```python
from build123d import *

# Parameters (mm, degrees)
BOSS_EXTRUDE1_DEPTH      = 6
BOSS_EXTRUDE1_DEPTH_BACK = 73
SKETCH1_W                = 60
SKETCH1_H                = 40
CUT_EXTRUDE2_DEPTH       = 10
SKETCH7_W                = 64
SKETCH7_H                = 44
SKETCH7_W_2              = 60
SKETCH7_H_2              = 40
BOSS_EXTRUDE2_DEPTH      = 11.2
SKETCH5_W                = 24
SKETCH5_H                = 3
CUT_EXTRUDE3_DEPTH       = 11.2
SKETCH8_W                = 24
SKETCH8_H                = 3
CUT_EXTRUDE4_DEPTH       = 11.2
FILLET1_R                = 5


with BuildPart() as part:
    # Sketch2 → Boss-Extrude1 (new, two sides: drawn at the far end of the back side and taken through both)
    with BuildSketch(Plane(origin=(18.941176471, 0, 0), x_dir=(0, 0, -1), z_dir=(1, 0, 0)).offset(-BOSS_EXTRUDE1_DEPTH_BACK)):
        with BuildLine():
            Line((34.764705882, 0), (-9.235294118, 0))
            add(Edge.make_bspline(
                [(-16.859042356, 8.803732274), (-16.71202536, 7.645123783), (-16.476121405, 6.983025742), (-15.665438552, 5.367344471), (-15.146819104, 4.569071681), (-14.219232142, 3.103782941), (-13.097173401, 1.202110064), (-10.958273151, -0.0861532), (-9.235294118, 0)],
                knots=[0.100936793, 0.100936793, 0.100936793, 0.100936793, 0.214701658, 0.247771225, 0.411203439, 0.4591999, 0.679739374, 1, 1, 1, 1], degree=3))
            Line((-16.859042356, 8.803732274), (-20.331201871, 8.363155033))
            Line((-20.331201871, 8.363155033), (-21.979605491, 8.153991509))
            ThreePointArc((-21.979605491, 8.153991509), (-22.976524971, 7.58463131), (-23.278855037, 6.477104328))
            Line((-23.278855037, 6.477104328), (-23.215915431, 5.981081541))
            ThreePointArc((-23.215915431, 5.981081541), (-22.646555232, 4.984162061), (-21.53902825, 4.681831995))
            Line((-21.53902825, 4.681831995), (-19.89062463, 4.890995519))
            Line((-19.89062463, 4.890995519), (-19.371936566, 4.956811088))
            add(Edge.make_bspline(
                [(-19.371936566, 4.956811088), (-19.299083809, 4.805602772), (-19.143543885, 4.495535048), (-18.861030136, 3.961180263), (-18.379944727, 3.117280646), (-17.808764188, 2.238291872), (-17.267901922, 1.360604939), (-16.505554516, 0.170581495), (-15.372861084, -1.167927692), (-13.787032793, -2.419221644), (-12.034516859, -3.186353681), (-10.648338067, -3.44710609), (-10.029136817, -3.492321417), (-9.829873201, -3.5)],
                knots=[0.220066507, 0.220066507, 0.220066507, 0.220066507, 0.244323833, 0.26858116, 0.317095812, 0.414125118, 0.511154423, 0.608183729, 0.705213035, 0.80224234, 0.899271646, 0.947786298, 0.970646745, 0.970646745, 0.970646745, 0.970646745], degree=3))
            Line((-9.829873201, -3.5), (-9.158730941, -3.5))
            Line((-9.158730941, -3.5), (34.688142706, -3.5))
            Line((34.688142706, -3.5), (35.359284966, -3.5))
            add(Edge.make_bspline(
                [(35.359284966, -3.5), (35.558548581, -3.492321417), (36.177749832, -3.44710609), (37.563928624, -3.186353681), (39.316444558, -2.419221644), (40.902272849, -1.167927692), (42.034966281, 0.170581495), (42.797313687, 1.360604939), (43.338175952, 2.238291872), (43.909356491, 3.117280646), (44.390441901, 3.961180263), (44.67295565, 4.495535048), (44.828495573, 4.805602772), (44.901348331, 4.956811088)],
                knots=[0.245720713, 0.245720713, 0.245720713, 0.245720713, 0.26858116, 0.317095812, 0.414125118, 0.511154423, 0.608183729, 0.705213035, 0.80224234, 0.899271646, 0.947786298, 0.972043625, 0.996300951, 0.996300951, 0.996300951, 0.996300951], degree=3))
            Line((44.901348331, 4.956811088), (45.420036395, 4.890995519))
            Line((45.420036395, 4.890995519), (47.068440015, 4.681831995))
            ThreePointArc((47.068440015, 4.681831995), (48.175966997, 4.984162061), (48.745327196, 5.981081541))
            Line((48.745327196, 5.981081541), (48.808266802, 6.477104328))
            ThreePointArc((48.808266802, 6.477104328), (48.505936735, 7.58463131), (47.509017256, 8.153991509))
            Line((47.509017256, 8.153991509), (45.860613636, 8.363155033))
            Line((45.860613636, 8.363155033), (42.388454121, 8.803732274))
            add(Edge.make_bspline(
                [(42.388454121, 8.803732274), (42.241437125, 7.645123783), (42.00553317, 6.983025742), (41.194850317, 5.367344471), (40.676230869, 4.569071681), (39.748643907, 3.103782941), (38.626585166, 1.202110064), (36.487684916, -0.0861532), (34.764705882, 0)],
                knots=[0.100936793, 0.100936793, 0.100936793, 0.100936793, 0.214701658, 0.247771225, 0.411203439, 0.4591999, 0.679739374, 1, 1, 1, 1], degree=3))
        make_face()
    extrude(amount=BOSS_EXTRUDE1_DEPTH + BOSS_EXTRUDE1_DEPTH_BACK)

    # Sketch1 → Cut-Extrude2 (cut)
    with BuildSketch(Plane(origin=(0, 0, 0), x_dir=(1, 0, 0), z_dir=(0, 1, 0))):
        with Locations((-13.058823529, 12.764705882)):
            Rectangle(SKETCH1_W, SKETCH1_H)
    extrude(amount=-CUT_EXTRUDE2_DEPTH, mode=Mode.SUBTRACT)

    # Sketch7 → Boss-Extrude2 (add)
    with BuildSketch(Plane.XZ.offset(3.5)):
        with Locations((-13.058823529, -12.764705882)):
            Rectangle(SKETCH7_W, SKETCH7_H)
        with Locations((-13.058823529, -12.764705882)):
            Rectangle(SKETCH7_W_2, SKETCH7_H_2, mode=Mode.SUBTRACT)
    extrude(amount=BOSS_EXTRUDE2_DEPTH)

    # Sketch5 → Cut-Extrude3 (cut)
    with BuildSketch(Plane(origin=(0, 7.29739461, 0.925955726), x_dir=(1, 0, 0), z_dir=(0, -0.9920455755956746, -0.12587921171125438))):
        with Locations((-33.058823529, 19.686118423)):
            Rectangle(SKETCH5_W, SKETCH5_H)
        with Locations((3.941176471, 19.686118423)):
            Rectangle(SKETCH5_W, SKETCH5_H)
    extrude(amount=-CUT_EXTRUDE3_DEPTH, mode=Mode.SUBTRACT)

    # Sketch8 → Cut-Extrude4 (cut)
    with BuildSketch(Plane(origin=(0, 13.957613838, -1.7710612), x_dir=(1, 0, 0), z_dir=(0, 0.9920455755956736, -0.12587921171126285))):
        with Locations((-33.058823529, 43.523881917)):
            Rectangle(SKETCH8_W, SKETCH8_H)
        with Locations((3.941176471, 43.523881917)):
            Rectangle(SKETCH8_W, SKETCH8_H)
    extrude(amount=-CUT_EXTRUDE4_DEPTH, mode=Mode.SUBTRACT)

    # Fillet1
    # the kernel refuses this fillet: 5 mm, written as the material it takes off along each edge
    with BuildSketch(Plane(origin=(18.941176471, 8.803732274, -42.388454121), x_dir=(0, -0.12587921171125008, -0.9920455755956751), z_dir=(-1, 0, 0))) as fillet1_piece_1:
        with BuildLine():
            CenterArc((4.027488586, 5), FILLET1_R, 201.320916369, 68.679083631)
            Line((-0.6303042, 3.182043355), (-0.723460056, 3.145684222))
            ThreePointArc((-0.723460056, 3.145684222), (-0.228216041, 1.608856089), (-0.1, -2.43e-07))
            Line((-0.1, -2.43e-07), (0, -0.1))
            Line((0, -0.1), (4.027488586, -0.1))
            Line((4.027488586, -0.1), (4.027488586, 0))
        make_face()
    extrude(amount=83.068721464, mode=Mode.SUBTRACT)
    with BuildSketch(Plane(origin=(18.941176471, 8.803732274, 16.859042356), x_dir=(0, -0.12587921171124858, 0.9920455755956752), z_dir=(-1, 0, 0))) as fillet1_piece_2:
        with BuildLine():
            CenterArc((4.027488586, -5), FILLET1_R, 90, 68.679083631)
            Line((-0.6303042, -3.182043355), (-0.723460056, -3.145684222))
            ThreePointArc((-0.723460056, -3.145684222), (-0.228216041, -1.608856089), (-0.1, 2.43e-07))
            Line((-0.1, 2.43e-07), (0, 0.1))
            Line((0, 0.1), (4.027488586, 0.1))
            Line((4.027488586, 0.1), (4.027488586, 0))
        make_face()
    extrude(amount=83.068721464, mode=Mode.SUBTRACT)
    with BuildSketch(Plane(origin=(18.941176471, 8.803732274, 16.859042356), x_dir=(0, -0.948678952181438, -0.31624080332545423), z_dir=(1, 0, 0))) as fillet1_piece_3:
        with BuildLine():
            CenterArc((4.12213797, -4.922259934), FILLET1_R, 100.116712127, 68.679083631)
            Line((-0.782566531, -3.950728279), (-0.880660621, -3.931297646))
            Line((-0.880660621, -3.931297646), (-0.09809409, 0.019430633))
            Line((-0.09809409, 0.019430633), (0.019430395, 0.098094137))
            ThreePointArc((0.019430395, 0.098094137), (1.622536562, -0.088744475), (3.226303182, 0.098445199))
            Line((3.226303182, 0.098445199), (3.24386857, 0))
        make_face()
    extrude(amount=16.068721464, mode=Mode.SUBTRACT)
    with BuildSketch(Plane(origin=(18.941176471, 8.803732274, -42.388454121), x_dir=(0, -0.12587921171125008, -0.9920455755956751), z_dir=(1, 0, 0))) as fillet1_piece_4:
        with BuildLine():
            CenterArc((4.027488586, -5), FILLET1_R, 90, 68.679083631)
            Line((-0.6303042, -3.182043355), (-0.723460056, -3.145684222))
            ThreePointArc((-0.723460056, -3.145684222), (-0.228216041, -1.608856089), (-0.1, 2.43e-07))
            Line((-0.1, 2.43e-07), (0, 0.1))
            Line((0, 0.1), (4.027488586, 0.1))
            Line((4.027488586, 0.1), (4.027488586, 0))
        make_face()
    extrude(amount=16.068721464, mode=Mode.SUBTRACT)


solid = part.part
```
Design review of the part built by this model. Coordinates are the model's own, in mm. A direction names the side the tool comes from. Coordinates: 2 decimals unless noted, no trailing zeros. Order: outer loops, then holes, each group sorted by start corner. A loop starts at its lowest first (then second) coordinate and runs counter-clockwise, first axis right, second up.
1) Take a section at A-A, the plane z = -31. Give the boundary of the cut face in (x, y), and give its area (3 significant figures).
2) Take a section at B-B, the plane y = -8. Give the boundary of the cut face in (x, z), and give its area (3 significant figures).
3) Mouldability with a two-part tool opening along X and no side actions: class faces 4 (the cylindrical face through (-14.01, 7.42, -42.87)), 5 (the flat face through (-43.059, -7, -13)), 6 (the flat face through (-45.059, -9, -13)), 7 (the flat face through (24.941, -0.2, -12.6)) as +X half, -X half, draft (parallel to the pull), parting line (faces both ways), or undercut.
4) For faces 1 (the flat face through (3.77, 6.61, 19.17)), 2 (the flat face through (16.941, -7, -13)), 3 (the flat face through (18.941, -9, -13)), list the 3-axis set-ups (+Z, -Z, +X, -X, +Y, -Y) from which the entire face can be reached by the end or side of a thin tool; tool diameter is ignored.
5) Wall thickness on line 1 along Z through (x, y) = (13, -8.25); line 2 along X through (y, z) = (-10, -10.5); line 3 along Z through (x, y) = (-43.5, -4.5): over which ranges is each line inside the solid? List them lowest first.
6) Take a section at C-C, the plane x = -44. State how many separate pieces and enclosed holes the cut face has, and give its area (3 significant figures).
7) Clearance check with flat-ended pins moving along their axes: pin 1 (4 mm diameter, centred on x = -24.5, y = -9.5, fed in from -Z); pin 2 (8 mm diameter, centred on y = -8, z = -13, fed in from +X); pin 3 (6 mm diameter, centred on x = -37.5, y = -2.5, fed in from +Z); pin 4 (22 mm diameter, centred on x = -0.5, z = -16, fed in from +Y). State where each tip first meets the part, or that it passes through.
Returned:
1. outline: (-54.06, -3.5) - (-45.06, -3.5) - (-45.06, -14.7) - (-43.06, -14.7) - (-43.06, 0) - (-54.06, 0) - close; (16.94, -14.7) - (18.94, -14.7) - (18.94, -3.5) - (24.94, -3.5) - (24.94, 0) - (16.94, 0) - close
1. area: 111 mm2
2. outline: (-45.06, -34.76) - (18.94, -34.76) - (18.94, 9.24) - (-45.06, 9.24) - close; hole (-43.06, -32.76) - (16.94, -32.76) - (16.94, 7.24) - (-43.06, 7.24) - close
2. area: 416 mm2
3. face 4: draft
3. face 5: undercut
3. face 6: -X half
3. face 7: +X half
4. face 1: none
4. face 2: +Y, -Y
4. face 3: +Z, -Z, +X, -Y
5. line 1: z = -34.76 to -32.76, 7.24 to 9.24
5. line 2: x = -45.06 to -43.06, 16.94 to 18.94
5. line 3: z = -34.76 to 9.24
6. separate pieces: 3
6. enclosed holes: 0
6. area: 744 mm2
7. pin 1: stops at z = -34.76
7. pin 2: stops at x = 18.94
7. pin 3: stops at z = 16.7
7. pin 4: passes through
